Geometry check sheet. Reference: the model listing, model coordinates, mm. A direction names the side the tool comes from. Give positions to 0.01 mm unless a question says otherwise; leave off trailing zeros. Loops run counter-clockwise (first coordinate to the right, second up) from the corner with the lowest first, then second, coordinate; pieces in that order, holes last. Notation, with made-up numbers: (16, -12.5) -> (21, -12.5) arc R24 cw to (21, 25.5) -> close; hole circle Ø10 at (35, 12.25). An arc over 180 degrees is marked (long way). Answer in a Markdown table with one row per item. Add a question column.
```python
from build123d import *

# Parameters (mm, degrees)
F0_W     = 30
F0_H     = 55
F0_R     = 2
F0_W_2   = 21.5
F0_H_2   = 28.5
F1_DEPTH = 1
F3_DEPTH = 36
F5_DEPTH = 5.001
F6_SIZE  = 5
F7_R     = 1


with BuildPart() as f1:
    # F0 (on Front) → F1 (new body)
    with BuildSketch(Plane.XZ):
        with Locations((-15, 27.5)):
            Rectangle(F0_W, F0_H)
        with Locations((-15, 7.5)):
            Circle(F0_R, mode=Mode.SUBTRACT)
        with Locations((-15, 27.5)):
            Rectangle(F0_W_2, F0_H_2, mode=Mode.SUBTRACT)
        with Locations((-15, 47.5)):
            Circle(F0_R, mode=Mode.SUBTRACT)
    extrude(amount=F1_DEPTH)

    # F2 (on face) → F3 (join)
    with BuildSketch(Plane.XZ.offset(1)):
        Polygon((0, 0), (0, 55), (-1, 55), (-1, -1), (4, -1), (4, 0), align=None)
    extrude(amount=F3_DEPTH)

    # F4 (on face) → F5 (cut, through all)
    with BuildSketch(Plane(origin=(-1, 0, 0), x_dir=(0, -1, 0), z_dir=(-1, 0, 0))):
        with BuildLine():
            ThreePointArc((21, 42.5), (19, 44.5), (17, 42.5))
            Line((17, 42.5), (17, 37.5))
            ThreePointArc((17, 37.5), (19, 35.5), (21, 37.5))
            Line((21, 37.5), (21, 42.5))
        make_face()
    extrude(amount=-F5_DEPTH, mode=Mode.SUBTRACT)

    # F6
    f6_edges = [f1.edges().sort_by_distance(p)[0] for p in [
        (-30, -0.5, 55),
        (-0.5, -37, 55),
        (-30, -0.5, 0),
    ]]
    chamfer(f6_edges, length=F6_SIZE)

    # F7
    f7_edges = [f1.edges().sort_by_distance(p)[0] for p in [
        (0, 0, 27.5),
        (-1, -19, -1),
    ]]
    fillet(f7_edges, radius=F7_R)


solid = f1.part
```
1. Sectioned sample at C-C (z = 39.5). Enter the section's corners in (x, y).
2. Sectioned sample at A-A (y = -19). Enter the section's corners in (x, z).
3. Sectioned sample at D-D (x = -19). Enter the section's corners in (y, z).
4. Sectioned sample at B-B (z = 47.5). Enter the section's corners in (x, y), plus the area to 3 significant figures.
5. Material ranges on L1, parallel to Z at x = -15, y = -0.7; L2, parallel to X at y = -24, z = 41.5, recorded low to high. Write a range as from..to.
6. Release check for a two-part mould opening along Y. For faces 6 (the face through (-3, -1, 28)), 7 (the face through (-0.5, -19, 35.5)), 8 (the face through (-3, 0, 28)) record: released by +Y, released by -Y, zero draft, split by the parting line, or undercut.
7. Access from +Z, -Z, +X, -X, +Y, -Y to the whole of each face (thin tool, end or side, straight path). Record for faces 1 (the face through (-0.5, -34.5, 52.5)), 2 (the face through (-1, -19, 28)), 3 (the face through (-27.5, -0.5, 2.5)), 4 (the face through (0, -19, 27)), 5 (the face through (-0.5, -19, 44.5)).
8. Gauge pin test, flat ends, axial feed: pin 1 Ø2.5 at (x, z) = (-15, 47.5) entering from -Y; pin 2 Ø8.5 at (x, z) = (-16, 16.5) entering from -Y; pin 3 Ø1.1 at (x, y) = (-16, -0.5) entering from -Z; pin 4 Ø1.5 at (y, z) = (-9, 26) entering from -X. Record the tip position at first contact, or that the pin passes through.
Response:
| question | item | result |
|---|---|---|
| 1 | outline | (-30, -1) -> (-25.75, -1) -> (-25.75, 0) -> (-30, 0) -> close; (-4.25, -1) -> (-1, -1) -> (-1, -17) -> (0, -17) -> (0, -1) arc R1 ccw to (-1, 0) -> (-4.25, 0) -> close; (-1, -37) -> (0, -37) -> (0, -21) -> (-1, -21) -> close |
| 2 | outline | (-1, 0) arc R1 ccw to (0, -1) -> (4, -1) -> (4, 0) -> (0, 0) -> (0, 35.5) -> (-1, 35.5) -> close; (-1, 44.5) -> (0, 44.5) -> (0, 55) -> (-1, 55) -> close |
| 3 | outline | (-1, 0) -> (0, 0) -> (0, 13.25) -> (-1, 13.25) -> close; (-1, 41.75) -> (0, 41.75) -> (0, 55) -> (-1, 55) -> close |
| 4 | outline | (-30, -1) -> (-17, -1) -> (-17, 0) -> (-30, 0) -> close; (-13, -1) -> (-1, -1) -> (-1, -37) -> (0, -37) -> (0, -1) arc R1 ccw to (-1, 0) -> (-13, 0) -> close |
| 4 | area | 61.8 mm2 |
| 5 | L1 | z = 0..5.5, 9.5..13.25, 41.75..45.5, 49.5..55 |
| 5 | L2 | x = -1..0 |
| 6 | face 6 | released by -Y |
| 6 | face 7 | undercut |
| 6 | face 8 | released by +Y |
| 7 | face 1 | +Z, +X, -X, -Y |
| 7 | face 2 | +Z, -Z, -X, -Y |
| 7 | face 3 | -Z, -X, +Y, -Y |
| 7 | face 4 | +Z, +X, +Y, -Y |
| 7 | face 5 | +X, -X |
| 8 | pin 1 | passes through |
| 8 | pin 2 | stops at y = -1 |
| 8 | pin 3 | stops at z = 0 |
| 8 | pin 4 | stops at x = -1 |
